The listing builds one solid part. Answer for the finished solid, in the listing's coordinates (mm). A direction names the side the tool comes from. Give positions to 0.01 mm unless a question says otherwise; leave off trailing zeros. Write each loop counter-clockwise with the first axis right and the second up, starting at its lowest first coordinate (ties: lowest second). Pieces come first, ordered by that corner, then holes.
```python
from build123d import *

# Parameters (mm, degrees)
SKETCH1_W           = 69.5
SKETCH1_H           = 82
BOSS_EXTRUDE1_DEPTH = 2
BOSS_EXTRUDE3_START = -2
BOSS_EXTRUDE3_DEPTH = 2
FILLET1_R           = 2


with BuildPart() as part:
    # Sketch1 → Boss-Extrude1 (new body)
    # profile 1 of 2: a face of its own
    with BuildSketch(Plane(origin=(0, 0, 0), x_dir=(1, 0, 0), z_dir=(0, 1, 0))):
        Rectangle(SKETCH1_W, SKETCH1_H)
        with BuildLine():
            ThreePointArc((7.602792708, -35), (5.602792708, -37), (3.602792708, -35))
            Line((3.602792708, -35), (-28.75, -35))
            Line((-28.75, -35), (-28.75, 33))
            ThreePointArc((-28.75, 33), (-30.164213562, 36.414213562), (-26.75, 35))
            Line((-26.75, 35), (26.75, 35))
            ThreePointArc((26.75, 35), (28.75, 37), (30.75, 35))
            ThreePointArc((30.75, 35), (30.164213562, 33.585786438), (28.75, 33))
            Line((28.75, 33), (28.75, -35))
            Line((28.75, -35), (7.602792708, -35))
        make_face(mode=Mode.SUBTRACT)
    # profile 2 of 2: a face of its own
    with BuildSketch(Plane(origin=(0, 0, 0), x_dir=(1, 0, 0), z_dir=(0, 1, 0))):
        with BuildLine():
            Line((-28.75, -35), (3.602792708, -35))
            ThreePointArc((3.602792708, -35), (5.602792708, -33), (7.602792708, -35))
            Line((7.602792708, -35), (28.75, -35))
            Line((28.75, -35), (28.75, 33))
            ThreePointArc((28.75, 33), (27.335786438, 33.585786438), (26.75, 35))
            Line((26.75, 35), (-26.75, 35))
            ThreePointArc((-26.75, 35), (-27.335786438, 33.585786438), (-28.75, 33))
            Line((-28.75, 33), (-28.75, -35))
        make_face()
    extrude(amount=BOSS_EXTRUDE1_DEPTH)

    # Sketch2 → Boss-Extrude3 (add)
    with BuildSketch(Plane(origin=(0, 2, 0), x_dir=(1, 0, 0), z_dir=(0, 1, 0)).offset(BOSS_EXTRUDE3_START)):
        with BuildLine():
            Line((47.602792708, -40.964572004), (34.75, -40.964572004))
            Line((34.75, -40.964572004), (34.75, -41))
            Line((34.75, -41), (-34.75, -41))
            Line((-34.75, -41), (-34.75, -40.964572004))
            Line((-34.75, -40.964572004), (-36.397207292, -40.964572004))
            Line((-36.397207292, -40.964572004), (-36.397207292, -37))
            ThreePointArc((-36.397207292, -37), (-38.397207292, -35), (-36.397207292, -33))
            Line((-36.397207292, -33), (-36.397207292, -29.035427996))
            Line((-36.397207292, -29.035427996), (-34.75, -29.035427996))
            Line((-34.75, -29.035427996), (-34.75, -25.680337555))
            Line((-34.75, -25.680337555), (-41.343372537, -25.680337555))
            Line((-41.343372537, -25.680337555), (-41.343372537, -44.319662445))
            Line((-41.343372537, -44.319662445), (52.548957953, -44.319662445))
            Line((52.548957953, -44.319662445), (52.548957953, -25.680337555))
            Line((52.548957953, -25.680337555), (34.75, -25.680337555))
            Line((34.75, -25.680337555), (34.75, -29.035427996))
            Line((34.75, -29.035427996), (47.602792708, -29.035427996))
            Line((47.602792708, -29.035427996), (47.602792708, -33))
            ThreePointArc((47.602792708, -33), (49.01700627, -33.585786438), (49.602792708, -35))
            ThreePointArc((49.602792708, -35), (49.01700627, -36.414213562), (47.602792708, -37))
            Line((47.602792708, -37), (47.602792708, -40.964572004))
        make_face()
        with BuildLine():
            ThreePointArc((7.602792708, -35), (5.602792708, -37), (3.602792708, -35))
            Line((3.602792708, -35), (-34.397207292, -35))
            ThreePointArc((-34.397207292, -35), (-34.487441, -35.593963558), (-34.75, -36.134331582))
            Line((-34.75, -36.134331582), (-34.75, -40.964572004))
            Line((-34.75, -40.964572004), (34.75, -40.964572004))
            Line((34.75, -40.964572004), (34.75, -35))
            Line((34.75, -35), (7.602792708, -35))
        make_face()
        with BuildLine():
            Line((-34.397207292, -35), (3.602792708, -35))
            ThreePointArc((3.602792708, -35), (5.602792708, -33), (7.602792708, -35))
            Line((7.602792708, -35), (34.75, -35))
            Line((34.75, -35), (34.75, -29.035427996))
            Line((34.75, -29.035427996), (-34.75, -29.035427996))
            Line((-34.75, -29.035427996), (-34.75, -33.865668418))
            ThreePointArc((-34.75, -33.865668418), (-34.487441, -34.406036442), (-34.397207292, -35))
        make_face()
        with BuildLine():
            Line((45.602792708, -35), (34.75, -35))
            Line((34.75, -35), (34.75, -40.964572004))
            Line((34.75, -40.964572004), (47.602792708, -40.964572004))
            Line((47.602792708, -40.964572004), (47.602792708, -37))
            ThreePointArc((47.602792708, -37), (46.188579146, -36.414213562), (45.602792708, -35))
        make_face()
        with BuildLine():
            Line((34.75, -29.035427996), (34.75, -35))
            Line((34.75, -35), (45.602792708, -35))
            ThreePointArc((45.602792708, -35), (46.188579146, -33.585786438), (47.602792708, -33))
            Line((47.602792708, -33), (47.602792708, -29.035427996))
            Line((47.602792708, -29.035427996), (34.75, -29.035427996))
        make_face()
        with BuildLine():
            Line((-34.75, -40.964572004), (-34.75, -36.134331582))
            ThreePointArc((-34.75, -36.134331582), (-35.466794256, -36.770404355), (-36.397207292, -37))
            Line((-36.397207292, -37), (-36.397207292, -40.964572004))
            Line((-36.397207292, -40.964572004), (-34.75, -40.964572004))
        make_face()
        with BuildLine():
            ThreePointArc((-36.397207292, -33), (-35.466794256, -33.229595645), (-34.75, -33.865668418))
            Line((-34.75, -33.865668418), (-34.75, -29.035427996))
            Line((-34.75, -29.035427996), (-36.397207292, -29.035427996))
            Line((-36.397207292, -29.035427996), (-36.397207292, -33))
        make_face()
    extrude(amount=BOSS_EXTRUDE3_DEPTH)

    # Fillet1
    fillet1_edges = [part.edges().sort_by_distance(p)[0] for p in [
        (34.75, 1, -41),
        (-34.75, 1, -41),
        (34.75, 1, 25.680337555),
        (52.548957953, 1, 25.680337555),
        (52.548957953, 1, 44.319662445),
        (-41.343372537, 1, 44.319662445),
        (-41.343372537, 1, 25.680337555),
        (-34.75, 1, 25.680337555),
    ]]
    fillet(fillet1_edges, radius=FILLET1_R)


solid = part.part
```
Item 1: A cutting plane is placed at A-A, the plane y = 0.3. Give the vertices of the cut face in (x, z).
Conclusion:
outline: (-41.34, 27.68) arc R2 ccw to (-39.34, 25.68) - (-36.75, 25.68) arc R2 cw to (-34.75, 23.68) - (-34.75, -39) arc R2 ccw to (-32.75, -41) - (32.75, -41) arc R2 ccw to (34.75, -39) - (34.75, 23.68) arc R2 cw to (36.75, 25.68) - (50.55, 25.68) arc R2 ccw to (52.55, 27.68) - (52.55, 42.32) arc R2 ccw to (50.55, 44.32) - (-39.34, 44.32) arc R2 ccw to (-41.34, 42.32) - close; hole (-34.75, 33.87) - (-34.75, 36.13) arc R2 ccw (long way) to start; hole circle Ø4 at (-28.75, -35); hole circle Ø4 at (5.6, 35); hole circle Ø4 at (28.75, -35); hole circle Ø4 at (47.6, 35)
Item 2: Determine the mould class of faces 6 (the face through (6.04, 0.99, 36.95)), 7 (the face through (44, 1, 25.68)), 8 (the face through (-40.74, 1.01, 43.75)) for opening direction Z: pulls with the +Z half, pulls with the -Z half, needs draft (parallel to the pull), parting line crosses it, or undercut.
Conclusion:
face 6: undercut
face 7: pulls with the -Z half
face 8: pulls with the +Z half
Item 3: Which of the six approach directions +Z, -Z, +X, -X, +Y, -Y give full straight-line access (tool end or side, diameter ignored) to faces 1 (the face through (-34.75, 1, 35)), 2 (the face through (0, 1, -41)), 3 (the face through (51.979, 1.014, 43.718)), 4 (the face through (34.75, 1, -7)), 5 (the face through (-34.75, 1, -7))?
Conclusion:
face 1: +Y, -Y
face 2: -Z, +X, -X, +Y, -Y
face 3: +Z, +X, +Y, -Y
face 4: -Z, +X, +Y, -Y
face 5: -Z, -X, +Y, -Y
Item 4: Each of these flat-tipped pins is pushed along its axis until it touches: P1, Ø4.5, axis at x = -28.75, z = -35, coming from the -Y side; P2, Ø1, axis at y = 1.5, z = -12.5, coming from the -X side; P3, Ø1, axis at x = 44.5, y = 1, coming from the -Z side. Where does it stop, or does it pass through?
Conclusion:
P1: stops at y = 0
P2: stops at x = -34.75
P3: stops at z = 25.68
Item 5: Consider probe 1 along X at (y, z) = (0.9, -35); probe 2 along X at (y, z) = (1.25, 35); probe 3 along Z at (x, y) = (-29, 1.9). Determine where each line is inside the solid, lowest interval first.
Conclusion:
probe 1: x = -34.75 to -30.75, -26.75 to 26.75, 30.75 to 34.75
probe 2: x = -41.34 to -38.4, -34.75 to 3.6, 7.6 to 45.6, 49.6 to 52.55
probe 3: z = -41 to -36.98, -33.02 to 44.32
Item 6: A cutting plane is placed at B-B, the plane z = 4.5. Give the vertices of the cut face in (x, y), plus the area to 3 significant figures.
Conclusion:
outline: (-34.75, 0) - (34.75, 0) - (34.75, 2) - (-34.75, 2) - close
area: 139 mm2
